```python
from build123d import *

# Parameters (mm, degrees)
EXTRUDE_1_DEPTH          = 4
EXTRUDE_START            = -4
SKETCH_3_W               = 23.208015554
SKETCH_3_H               = 15.560947598
EXTRUDE_2_DEPTH          = 4
SKETCH_7_W               = 7
SKETCH_7_H               = 15
EXTRUDE_3_DEPTH          = 23.208015554
CUT_EXTRUDE_6_DEPTH      = 25
SKETCH_5_R               = 1.35
SKETCH_5_R_2             = 1.6
CUT_EXTRUDE_2_DEPTH      = 41
FILLET_1_R               = 1
CUT_EXTRUDE_9_DEPTH      = 132.632440775
CUT_EXTRUDE_9_DEPTH_BACK = 132.632440775
SKETCH_16_R              = 17.5
EXTRUDE_5_DEPTH          = 4
FILLET_8_R               = 1
FILLET_10_R              = 1
FILLET_12_R              = 1
FILLET_13_R              = 1.5
RIB_1_REACH              = 137.852
SKETCH_19_WALL_W         = 283.05422189
SKETCH_19_WALL_H         = 10
FILLET_START             = -15.424467696
FILLET_14_DEPTH          = 30.848935392
FILLET_START_2           = -12.604007877
FILLET_14_2_DEPTH        = 25.208015654
FILLET_START_3           = -30.058809371
FILLET_14_3_DEPTH        = 2.058809371
FILLET_15_R              = 5


with BuildPart() as part:
    # 草图2 → 凸台-拉伸1 (new body)
    with BuildSketch(Plane(origin=(-34.058809371, 0, 0), x_dir=(0, 0, -1), z_dir=(1, 0, 0))):
        with BuildLine():
            Line((17.500319827, 130.276008038), (17.500319827, 126.359600173))
            ThreePointArc((17.500319827, 126.359600173), (17.374404969, 125.661169877), (17.012514948, 125.050682332))
            ThreePointArc((17.012514948, 125.050682332), (15.910222403, 123.866105461), (14.725645532, 122.763812916))
            ThreePointArc((14.725645532, 122.763812916), (14.115157987, 122.401922895), (13.416727692, 122.276008038))
            Line((13.416727692, 122.276008038), (8.570604361, 122.276008038))
            Line((8.570604361, 122.276008038), (-4.829395639, 122.276008038))
            Line((-4.829395639, 122.276008038), (-13.416088038, 122.276008038))
            ThreePointArc((-13.416088038, 122.276008038), (-14.114518334, 122.401922895), (-14.725005879, 122.763812916))
            ThreePointArc((-14.725005879, 122.763812916), (-15.90958275, 123.866105461), (-17.011875295, 125.050682332))
            ThreePointArc((-17.011875295, 125.050682332), (-17.373765316, 125.661169877), (-17.499680173, 126.359600173))
            Line((-17.499680173, 126.359600173), (-17.499680173, 130.276008038))
            Line((-17.499680173, 130.276008038), (17.500319827, 130.276008038))
        make_face()
    extrude(amount=EXTRUDE_1_DEPTH)

    # 草图3 → 凸台-拉伸2 (add)
    with BuildSketch(Plane(origin=(-30.058809371, 0, 0), x_dir=(0, 0, -1), z_dir=(1, 0, 0)).offset(EXTRUDE_START)):
        with Locations((0, 114.495534239)):
            Rectangle(SKETCH_3_W, SKETCH_3_H)
    extrude(amount=EXTRUDE_2_DEPTH)

    # 草图7 → 凸台-拉伸3 (add)
    with BuildSketch(Plane.XY.offset(11.604007777)):
        with Locations((-26.558809371, 114.21506044)):
            Rectangle(SKETCH_7_W, SKETCH_7_H)
    extrude(amount=-EXTRUDE_3_DEPTH)

    # 草图11 → 切除-拉伸6 (cut)
    with BuildSketch(Plane.XY.offset(11.604007777)):
        with BuildLine():
            Line((-17.260737948, 105.57071884), (-17.822335609, 118.157865003))
            ThreePointArc((-17.822335609, 118.157865003), (-20.746096987, 118.264862867), (-23.654216554, 118.585284033))
            ThreePointArc((-23.654216554, 118.585284033), (-24.615393694, 118.539747196), (-25.488172243, 118.134540208))
            ThreePointArc((-25.488172243, 118.134540208), (-28.620362377, 115.459397112), (-31.295505473, 112.327206978))
            ThreePointArc((-31.295505473, 112.327206978), (-31.700712461, 111.454428429), (-31.746249298, 110.493251289))
            ThreePointArc((-31.746249298, 110.493251289), (-31.523200675, 108.69967015), (-31.381401894, 106.897844106))
            ThreePointArc((-31.381401894, 106.897844106), (-31.32637065, 105.4380129), (-31.324682737, 103.977145782))
            Line((-31.324682737, 103.977145782), (-17.260737948, 105.57071884))
        make_face()
    extrude(amount=-CUT_EXTRUDE_6_DEPTH, mode=Mode.SUBTRACT)

    # 草图5 → 切除-拉伸2 (cut)
    with BuildSketch(Plane(origin=(-30.058809371, 0, 0), x_dir=(0, 0, -1), z_dir=(1, 0, 0))):
        with Locations(Location((-14.318592493, 125.457095719, 0), (0, 0, 90))):
            Circle(SKETCH_5_R)
        with Locations(Location((14.319232146, 125.457095719, 0), (0, 0, 90))):
            Circle(SKETCH_5_R_2)
    extrude(amount=-CUT_EXTRUDE_2_DEPTH, mode=Mode.SUBTRACT)

    # 圆角1
    fillet_1_edges = [part.edges().sort_by_distance(p)[0] for p in [
        (-32.058809371, 122.276008038, -11.604007777),
    ]]
    fillet(fillet_1_edges, radius=FILLET_1_R)
    fillet_1_2_edges = [part.edges().sort_by_distance(p)[0] for p in [
        (-32.058809371, 122.276008038, 11.604007777),
    ]]
    fillet(fillet_1_2_edges, radius=FILLET_1_R)

    # 草图16 → 切除-拉伸9 (cut, two sides: drawn at the far end of the back side and taken through both)
    with BuildSketch(Plane(origin=(-30.058809371, 0, 0), x_dir=(0, 0, -1), z_dir=(1, 0, 0)).offset(-CUT_EXTRUDE_9_DEPTH_BACK)):
        with Locations((22.000319827, 103.276008038)):
            Circle(SKETCH_16_R)
        with Locations((-21.999680173, 103.276008038)):
            Circle(SKETCH_16_R)
    extrude(amount=CUT_EXTRUDE_9_DEPTH + CUT_EXTRUDE_9_DEPTH_BACK, mode=Mode.SUBTRACT)

    # 草图17 → 凸台-拉伸5 (add)
    with BuildSketch(Plane(origin=(-30.058809371, 0, 0), x_dir=(0, 0, -1), z_dir=(1, 0, 0)).offset(EXTRUDE_START)):
        with BuildLine():
            Line((-12.604007777, 122.276008038), (-13.416088038, 122.276008038))
            ThreePointArc((-13.416088038, 122.276008038), (-14.114518334, 122.401922895), (-14.725005879, 122.763812916))
            ThreePointArc((-14.725005879, 122.763812916), (-15.90958275, 123.866105461), (-17.011875295, 125.050682332))
            ThreePointArc((-17.011875295, 125.050682332), (-17.373765316, 125.661169877), (-17.499680173, 126.359600173))
            Line((-17.499680173, 126.359600173), (-17.499680173, 130.276008038))
            Line((-17.499680173, 130.276008038), (-17.999680173, 130.276008038))
            Line((-17.999680173, 130.276008038), (-17.999680173, 129.776008038))
            Line((-17.999680173, 129.776008038), (-17.999680173, 126.359600173))
            ThreePointArc((-17.999680173, 126.359600173), (-17.842286602, 125.486562303), (-17.389924076, 124.723452872))
            ThreePointArc((-17.389924076, 124.723452872), (-16.263136141, 123.512552071), (-15.052235339, 122.385764135))
            ThreePointArc((-15.052235339, 122.385764135), (-14.289125908, 121.93340161), (-13.416088038, 121.776008038))
            Line((-13.416088038, 121.776008038), (-12.604007777, 121.776008038))
            ThreePointArc((-12.604007777, 121.776008038), (-12.48056994, 121.760531619), (-12.364773606, 121.71506044))
            Line((-12.364773606, 121.71506044), (-11.705546321, 121.71506044))
            ThreePointArc((-11.705546321, 121.71506044), (-12.074410006, 122.124256941), (-12.604007777, 122.276008038))
        make_face()
    extrude_5 = extrude(amount=EXTRUDE_5_DEPTH)

    # 镜向1: 凸台-拉伸5 across plane
    add(extrude_5.mirror(Plane.XY))

    # 圆角8
    fillet_8_edges = [part.edges().sort_by_distance(p)[0] for p in [
        (-30.284407251, 117.353177347, -11.604007777),
        (-30.284113568, 117.353649723, 11.604007777),
    ]]
    fillet(fillet_8_edges, radius=FILLET_8_R)

    # 圆角10
    fillet_10_edges = [part.edges().sort_by_distance(p)[0] for p in [
        (-30.058809371, 130.276008038, 0),
    ]]
    fillet(fillet_10_edges, radius=FILLET_10_R)

    # 圆角12
    fillet_12_edges = [part.edges().sort_by_distance(p)[0] for p in [
        (-31.371585595, 106.71506044, -0.000319827),
        (-34.058809371, 106.71506044, -0.000319827),
    ]]
    fillet(fillet_12_edges, radius=FILLET_12_R)

    # 圆角13
    fillet_13_edges = [part.edges().sort_by_distance(p)[0] for p in [
        (-23.058809371, 121.71506044, 0),
        (-23.058809371, 118.502104481, 0),
    ]]
    fillet(fillet_13_edges, radius=FILLET_13_R)

    # 草图19 wall → 筋1 (add, up to next)
    with BuildSketch(Plane(origin=(-27.308809371, 125.495534239, 0), x_dir=(0.588250674462, -0.808678640744, 0), z_dir=(0.808678640744, 0.588250674462, 0)), mode=Mode.PRIVATE) as rib_1_sk1:
        Rectangle(SKETCH_19_WALL_W, SKETCH_19_WALL_H)
    rib_1_tool1 = extrude(rib_1_sk1.sketch, amount=-RIB_1_REACH, mode=Mode.PRIVATE) - part.part
    add(rib_1_tool1.solids().sort_by_distance((-27.308809371, 125.495534239, 0))[0])

    # 圆角14: read off the stored shape, not the designer's step
    # 圆角14 outline → 圆角14 (add)
    with BuildSketch(Plane.XY.offset(FILLET_START)):
        with BuildLine():
            Line((-30.058809371, 121.776008038), (-29.402583406, 121.776008038))
            ThreePointArc((-29.402583406, 121.776008038), (-29.878496517, 122.142248968), (-30.058809371, 122.71506044))
            Line((-30.058809371, 122.71506044), (-30.058809371, 121.776008038))
        make_face()
    extrude(amount=FILLET_14_DEPTH)

    # Fillet 14 2 outline → Fillet 14 2 (add)
    with BuildSketch(Plane.XY.offset(FILLET_START_2)):
        with BuildLine():
            Line((-30.058809371, 121.71506044), (-29.058809371, 121.71506044))
            ThreePointArc((-29.058809371, 121.71506044), (-29.233376834, 121.730415224), (-29.402583406, 121.776008038))
            Line((-29.402583406, 121.776008038), (-30.058809371, 121.776008038))
            Line((-30.058809371, 121.776008038), (-30.058809371, 121.71506044))
        make_face()
    extrude(amount=FILLET_14_2_DEPTH)

    # Fillet 14 3 outline → Fillet 14 3 (cut)
    with BuildSketch(Plane.YZ.offset(FILLET_START_3)):
        with BuildLine():
            ThreePointArc((121.71506044, 12.364773606), (121.760531619, 12.48056994), (121.776008038, 12.604007777))
            Line((121.776008038, 12.604007777), (121.71506044, 12.604007777))
            Line((121.71506044, 12.604007777), (121.71506044, 12.364773606))
        make_face()
        with BuildLine():
            ThreePointArc((121.776008038, 13.416088038), (121.93340161, 14.289125908), (122.385764135, 15.052235339))
            ThreePointArc((122.385764135, 15.052235339), (122.549406884, 15.23924095), (122.715060489, 15.424467652))
            Line((122.715060489, 15.424467652), (121.776008038, 15.424467696))
            Line((121.776008038, 15.424467696), (121.776008038, 13.416088038))
        make_face()
        with BuildLine():
            ThreePointArc((122.385764135, -15.052235339), (121.93340161, -14.289125908), (121.776008038, -13.416088038))
            Line((121.776008038, -13.416088038), (121.776008038, -15.424467696))
            Line((121.776008038, -15.424467696), (122.715060489, -15.424467652))
            ThreePointArc((122.715060489, -15.424467652), (122.549406884, -15.23924095), (122.385764135, -15.052235339))
        make_face()
        with BuildLine():
            Line((121.71506044, -12.604007877), (121.776008038, -12.604007777))
            ThreePointArc((121.776008038, -12.604007777), (121.760531619, -12.48056994), (121.71506044, -12.364773606))
            Line((121.71506044, -12.364773606), (121.71506044, -12.604007877))
        make_face()
    extrude(amount=FILLET_14_3_DEPTH, mode=Mode.SUBTRACT)

    # 圆角15
    fillet_15_edges = [part.edges().sort_by_distance(p)[0] for p in [
        (-30.058809371, 129.276008038, 0),
        (-24.558809371, 121.71506044, 0),
    ]]
    fillet(fillet_15_edges, radius=FILLET_15_R)


solid = part.part
```
Part model, mm, in its own coordinate system. A direction names the side the tool comes from. Give positions to 0.01 mm unless a question says otherwise; leave off trailing zeros. Loops run counter-clockwise (first coordinate to the right, second up) from the corner with the lowest first, then second, coordinate; pieces in that order, holes last. Notation, with made-up numbers: M -39,82 L 6,82 A21 ccw 6,118 Z; hole C 86.5,43.25 d8. An arc over 180 degrees is marked long. Return JSON: item names as keys, results as strings.
1) Pull direction Y, two halves, no side cores. Call faces 1 (the face through (-32.09, 123.53, 16.28)), 2 (the face through (-31.697, 111.468, 0.098)), 3 (the face through (-27, 121.715, -8)): released by +Y, released by -Y, zero draft, split by the parting line, or undercut.
Calculated:
{"face 1": "released by -Y", "face 2": "undercut", "face 3": "released by +Y"}
2) Saw through at A-A, the plane y = 128. List the corners of the cut face in (x, z), then the cut area to 3 significant figures.
Calculated:
{"outline": "M -34.06,-18 L -30.06,-18 L -30.06,-5 L -29.13,-5 L -29.13,5 L -30.06,5 L -30.06,18 L -34.06,18 Z", "area": "153 mm2"}
3) Drill centre lines: line 1 (Z direction, x = -33, y = 125.5); line 2 (Z direction, x = -33, y = 118); line 3 (X direction, y = 115, z = -7.5). Where is each one in solid material? Low to high.
Calculated:
{"line 1": "z = -17.85 to -15.92, -12.72 to 12.97, 15.67 to 17.85", "line 2": "z = -11.6 to 11.6", "line 3": "x = -34.06 to -29.07"}
4) Flat gauge pins, fed straight in: pin 1 Ø5 at (y, z) = (127.5, 10.5) entering from +X; pin 2 Ø1.5 at (x, z) = (-30.5, 0) entering from -Y; pin 3 Ø4 at (x, z) = (-25.5, 7.5) entering from -Y; pin 4 Ø3 at (y, z) = (125.46, -14.32) entering from +X. Where does each tip first touch, or does it go through?
Calculated:
{"pin 1": "stops at x = -30.06", "pin 2": "stops at y = 112.39", "pin 3": "stops at y = 116.52", "pin 4": "passes through"}
5) Saw through at B-B, the plane x = -27.5. List the corners of the cut face in (y, z).
Calculated:
{"outline": "M 116.52,-10.56 A17.5 cw 117.06,-11.22 A1 ccw 117.85,-11.6 L 121.28,-11.6 A1 cw 121.72,-11.71 L 121.72,-5 L 125.76,-5 L 125.76,5 L 121.72,5 L 121.72,11.71 A1 cw 121.28,11.6 L 117.85,11.6 A1 ccw 117.06,11.22 A17.5 cw 116.52,10.56 Z"}
6) 3-axis set-ups, long thin cutter, end or side, ignore diameter. For faces 4 (the face through (-29, 120, -11.604)), 5 (the face through (-29, 120, 11.604)), 6 (the face through (-28, 125, 5)), 7 (the face through (-30.059, 126, -12)): which of +Z, -Z, +X, -X, +Y, -Y reach the whole face in a straight line?
Calculated:
{"face 4": "-Z, +X, -X, -Y", "face 5": "+Z, +X, -X, -Y", "face 6": "+Z, +X, +Y", "face 7": "-Z, +X, +Y"}
